Verification items for the finished model (mm, model axes). Round coordinates to 2 decimals unless told otherwise and drop trailing zeros. Order: outer loops, then holes, each group sorted by start corner. A loop starts at its lowest first (then second) coordinate and runs counter-clockwise, first axis right, second up. Notation, with made-up numbers: (21.25, 59.25) -> (73.25, 59.25) arc R34 cw to (73.25, 97.25) -> close; hole circle Ø5 at (63.5, 81.5). An arc over 180 degrees is marked (long way). Return JSON: item names as keys, results as strings. Group by question number.
Item 1: Depth check by flat-ended pin: pin 1 Ø2 at (y, z) = (-93.5, 6) entering from +X; pin 2 Ø4 at (y, z) = (-108.5, 4) entering from +X; pin 3 Ø1 at (y, z) = (-133, 5.5) entering from -X. Enter the tip coordinate at first touch or a pass-through.
Item 2: Sectioned sample at A-A on z = 4. Record the cut outline in (x, y).
Item 3: Scan lines: probe 1 along X at (y, z) = (-36, 6.5); probe 2 along X at (y, z) = (33, 7.25); probe 3 along Y at (x, z) = (-190, 7.25). Record each from-to range of solid material in increasing order. Write a range as from..to.
Item 4: Sectioned sample at B-B on y = 18.5. Record the cut outline in (x, z), plus the area to 3 significant figures.
Item 5: Sectioned sample at C-C on x = -128.5. Record the cut outline in (y, z).
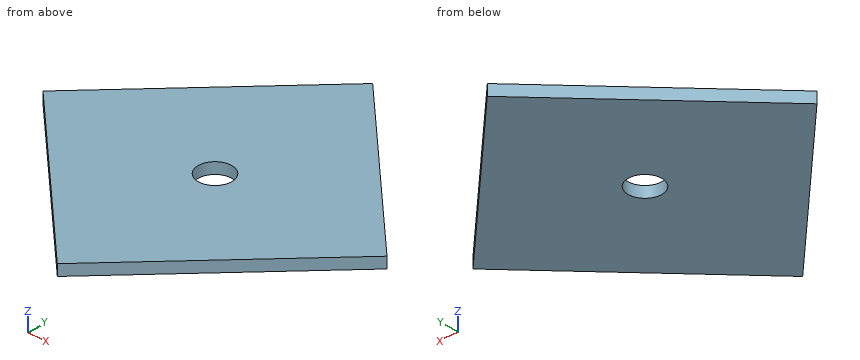
Autodesk Inventor part; units mm, degrees
ref_plane "YZ Plane" through (0, 0, 0) normal (1, 0, 0) x (0, 1, 0)
ref_plane "XZ Plane" through (0, 0, 0) normal (0, 1, 0) x (-1, 0, 0)
ref_plane "XY Plane" through (0, 0, 0) normal (0, 0, 1) x (1, 0, 0)
sketch "Sketch1" plane through (0, 0, 0) normal (0, 0, 1) x (1, 0, 0)
  line L0 (-46.0933, 91.1044) -> (-62.0933, 91.1044)
  line L1 (-54.0933, 118.5442) -> (-209.6568, -37.0193)
  line L2 (-209.6568, -37.0193) -> (-54.0933, -192.5828)
  line L3 (-54.0933, -192.5828) -> (101.4702, -37.0193)
  line L4 (101.4702, -37.0193) -> (-54.0933, 118.5442)
  line L5 (-54.0933, 91.1044) -> (165.9067, 91.1044) construction
  line L6 (-25.3821, 79.8544) -> (-25.3821, 89.8544)
  line L7 (-82.7831, 89.8544) -> (-82.7831, 79.8544)
  line L8 (-54.0933, 91.1044) -> (-54.0933, 151.1044)
  line L9 (-82.7831, 89.8544) -> (-54.0933, 118.5442)
  line L10 (-82.7831, 89.8544) -> (-42.2096, 89.8544) construction
  point P0 (0, 0)
  dimension "d0" = 220
  dimension "d1" = 135
  dimension "d2" = 220
  dimension "d3" = 60
  dimension "d4" = 45
extrude "Extrusion1" add sketch "Sketch1" along normal blind 10
sketch "Sketch2" plane through (0, 0, 0) normal (0, 0, -1) x (-1, 0, 0)
  line L0 (209.6568, -37.0193) -> (54.0933, -192.5828)
  line L1 (54.0933, 118.5442) -> (209.6568, -37.0193)
  line L2 (-101.4702, -37.0193) -> (54.0933, 118.5442)
  line L3 (54.0933, -192.5828) -> (-101.4702, -37.0193)
  line L4 (-101.4702, -37.0193) -> (209.6568, -37.0193)
  line L5 (54.0933, -192.5828) -> (54.0933, 118.5442)
  line L6 (74.0933, -3.2956) -> (34.0933, -3.2956)
  line L7 (34.0933, 39.0692) -> (74.0933, 39.0692)
  line L8 (74.0933, 39.0692) -> (74.0933, -3.2956)
  line L9 (74.0933, -3.2956) -> (34.0933, -3.2956)
  line L10 (34.0933, -3.2956) -> (34.0933, 39.0692)
  point P0 (0, 0)
sketch "Sketch3" plane through (0, 0, 0) normal (0, 0, -1) x (-1, 0, 0)
  line L0 (-101.4702, -37.0193) -> (209.6568, -37.0193)
  line L1 (54.0933, -192.5828) -> (54.0933, 118.5442)
  circle A0 centre (54.0933, -37.0193) radius 15.2178
  point P0 (0, 0)
extrude "Extrusion2" cut sketch "Sketch3" against normal blind 10
properties part number "Template220"
Recorded:
{
 "1": {"pin 1": "x = 45.99", "pin 2": "x = 31.99", "pin 3": "x = -114.18"},
 "2": {"outline": "(-209.66, -37.02) -> (-54.09, -192.58) -> (101.47, -37.02) -> (-54.09, 118.54) -> close; hole circle Ø30.44 at (-54.09, -37.02)"},
 "3": {"probe 1": "-208.64..-69.28, -38.91..100.45", "probe 2": "-139.64..31.45", "probe 3": "-56.68..-17.36"},
 "4": {"outline": "(-154.14, 0) -> (45.95, 0) -> (45.95, 10) -> (-154.14, 10) -> close", "area": "2,000 mm²"},
 "5": {"outline": "(-118.18, 0) -> (44.14, 0) -> (44.14, 10) -> (-118.18, 10) -> close"}
}
